Here's how the part is built. I have some questions about the finished solid (model axes, mm). A direction names the side the tool comes from. Round coordinates to 2 decimals unless told otherwise and drop trailing zeros. Write each loop counter-clockwise with the first axis right and the second up, starting at its lowest first coordinate (ties: lowest second). Pieces come first, ordered by that corner, then holes. Notation, with made-up numbers: (52, -9) - (79, -9) arc R11 cw to (79, -5) - close; hole circle Ø3 at (66.25, -25). An arc over 180 degrees is marked (long way). One line per question, with ' | ' between items. Start each with the question number.
(1) Imagine slicing it at A-A (x = -119.5). Write out the boundary of the cut face in (y, z).
(2) Imagine slicing it at C-C (x = 116.5). Write out the boundary of the cut face in (y, z).
(3) If I drill on L1, parallel to Z at x = -88.5, y = -356.5; L2, parallel to X at y = -338, z = -64.5, over which ranges is the centre line in solid material (lowest first)?
(4) Imagine slicing it at D-D (z = -74). Write out the boundary of the cut face in (x, y).
(5) Thinking about a two-plate mould opening in Z: for faces 3 (the flat face through (2, -270, 152.4)), 4 (the cylindrical face through (148.58, -173.73, -148.78)), 5 (the flat face through (2, -270, -146.05)), which applies, pulls with the +Z half, pulls with the -Z half, needs draft (parallel to the pull), parting line crosses it, or undercut?
(6) For faces 1 (the flat face through (146.05, -175, 2)), 2 (the flat face through (152.4, -172, -2)), which set-ups out of +Z, -Z, +X, -X, +Y, -Y let a thin tool reach every point of the face, with its end or its side?
(7) Imagine slicing it at B-B (y = -240). Write out the boundary of the cut face in (x, z), plus the area to 3 significant figures.
from build123d import *

# Parameters (mm, degrees)
F1_DEPTH = 444.5
F3_DEPTH = 304.801


with BuildPart() as f1:
    # F0 (on Front) → F1 (new body)
    with BuildSketch(Plane.XZ):
        with BuildLine():
            Line((-139.7, -152.4), (139.7, -152.4))
            ThreePointArc((139.7, -152.4), (148.6802561211, -148.6802561211), (152.4, -139.7))
            Line((152.4, -139.7), (152.4, 139.7))
            ThreePointArc((152.4, 139.7), (148.6802561211, 148.6802561211), (139.7, 152.4))
            Line((139.7, 152.4), (-139.7, 152.4))
            ThreePointArc((-139.7, 152.4), (-148.6802561211, 148.6802561211), (-152.4, 139.7))
            Line((-152.4, 139.7), (-152.4, -139.7))
            ThreePointArc((-152.4, -139.7), (-148.6802561211, -148.6802561211), (-139.7, -152.4))
        make_face()
        with BuildLine():
            Line((-139.7, 146.05), (139.7, 146.05))
            ThreePointArc((139.7, 146.05), (144.1901280605, 144.1901280605), (146.05, 139.7))
            Line((146.05, 139.7), (146.05, -139.7))
            ThreePointArc((146.05, -139.7), (144.1901280605, -144.1901280605), (139.7, -146.05))
            Line((139.7, -146.05), (-139.7, -146.05))
            ThreePointArc((-139.7, -146.05), (-144.1901280605, -144.1901280605), (-146.05, -139.7))
            Line((-146.05, -139.7), (-146.05, 139.7))
            ThreePointArc((-146.05, 139.7), (-144.1901280605, 144.1901280605), (-139.7, 146.05))
        make_face(mode=Mode.SUBTRACT)
    extrude(amount=F1_DEPTH)

    # F2 (on face) → F3 (cut, through all)
    with BuildSketch(Plane.XY.offset(152.4)):
        Polygon((-139.7, -444.5), (139.7, -444.5), (139.7, -352.4012237684), (-139.7, -440.4957053812), align=None)
        Polygon((139.7, -444.5), (152.4, -444.5), (152.4, -348.3969291497), (139.7, -352.4012237684), align=None)
        Polygon((-152.4, -444.5), (-139.7, -444.5), (-139.7, -440.4957053812), align=None)
        Polygon((139.7, -8.8926357353), (139.7, 0), (-139.7, 0), (-139.7, -204.5306219111), align=None)
        Polygon((-139.7, -204.5306219111), (-139.7, 0), (-152.4, 0), (-152.4, -213.4232576463), align=None)
        Polygon((139.7, -8.8926357353), (152.4, 0), (139.7, 0), align=None)
        Polygon((-152.4, -444.5), (-139.7, -440.4957053812), (-139.7, -204.5306219111), (-152.4, -213.4232576463), align=None)
    extrude(amount=-F3_DEPTH, mode=Mode.SUBTRACT)


solid = f1.part
Check sheet entries:
1) outline: (-434.13, -152.4) - (-190.39, -152.4) - (-190.39, -146.05) - (-434.13, -146.05) - close; (-434.13, 146.05) - (-190.39, 146.05) - (-190.39, 152.4) - (-434.13, 152.4) - close
2) outline: (-359.72, -152.4) - (-25.14, -152.4) - (-25.14, -146.05) - (-359.72, -146.05) - close; (-359.72, 146.05) - (-25.14, 146.05) - (-25.14, 152.4) - (-359.72, 152.4) - close
3) L1: -152.4 to -146.05, 146.05 to 152.4 | L2: 146.05 to 152.4
4) outline: (146.05, -350.4) - (152.4, -348.4) - (152.4, 0) - (146.05, -4.45) - close
5) face 3: pulls with the +Z half | face 4: pulls with the -Z half | face 5: undercut
6) face 1: -X, +Y, -Y | face 2: +Z, -Z, +X, +Y, -Y
7) outline: (-139.7, -152.4) - (139.7, -152.4) arc R12.7 ccw to (152.4, -139.7) - (152.4, 139.7) arc R12.7 ccw to (139.7, 152.4) - (-139.7, 152.4) - (-139.7, 146.05) - (139.7, 146.05) arc R6.35 cw to (146.05, 139.7) - (146.05, -139.7) arc R6.35 cw to (139.7, -146.05) - (-139.7, -146.05) - close | area: 5,510 mm^2
